Verification items for this drawing (mm, ordinates from the low corner). A direction names the side the tool comes from. Coordinates: 2 decimals unless noted, no trailing zeros. Order: outer loops, then holes, each group sorted by start corner. A loop starts at its lowest first (then second) coordinate and runs counter-clockwise, first axis right, second up.
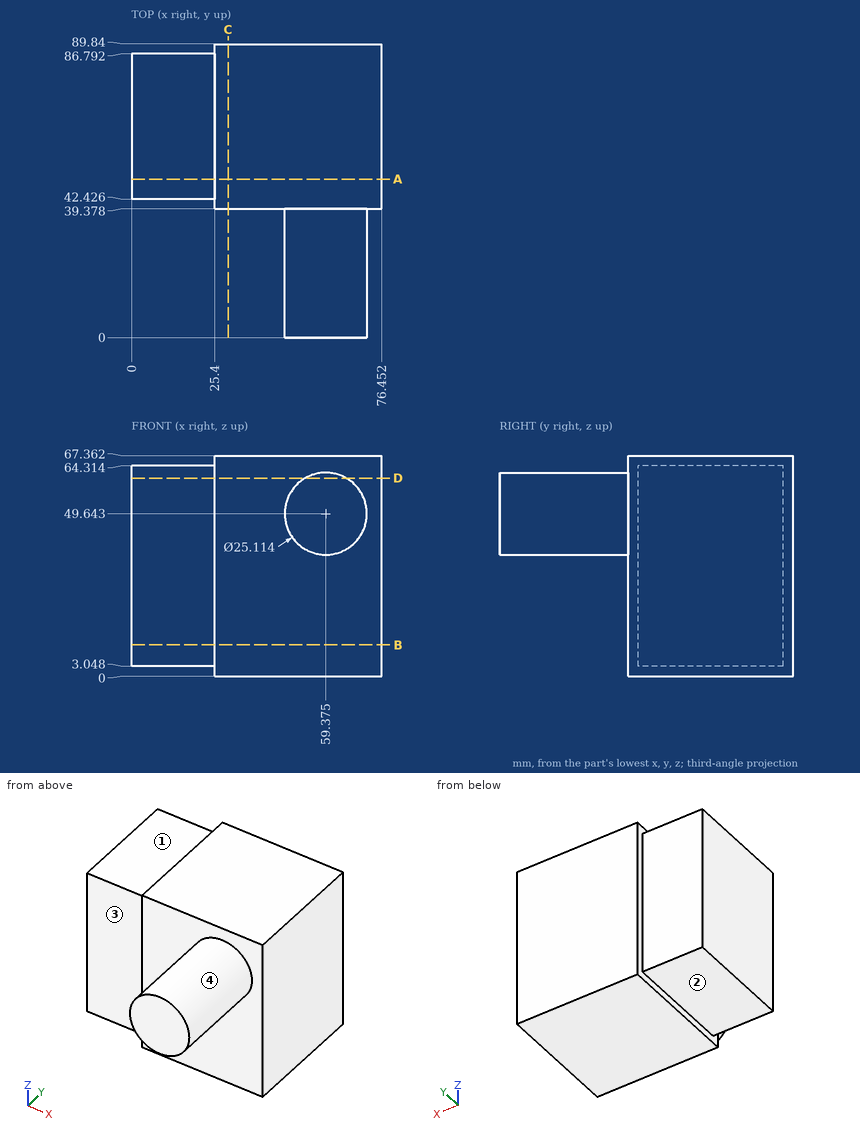
(1) Go/stop test with flat-tipped pins: P1, Ø8, axis at x = 42, y = 73, coming from the -Z side; P2, Ø7.5, axis at x = 12, z = 30, coming from the +Y side; P3, Ø3, axis at x = 38.5, z = 21.5, coming from the -Y side; P4, Ø7.5, axis at x = 14, z = 49, coming from the -Y side. Record where each tip stops, or that it passes through.
Filled in:
P1: stops at z = 0
P2: stops at y = 86.79
P3: stops at y = 39.38
P4: stops at y = 42.43
(2) Cross-section at D-D (z = 60.5). Enter the section's corners in (x, y) (1 decimal), and give its area (3 significant figures).
Filled in:
outline: (0, 42.4) - (25.4, 42.4) - (25.4, 39.4) - (53.1, 39.4) - (53.1, 0) - (65.7, 0) - (65.7, 39.4) - (76.5, 39.4) - (76.5, 89.8) - (25.4, 89.8) - (25.4, 86.8) - (0, 86.8) - close
area: 4,200 mm2
(3) Cross-section at A-A (y = 48.5). Enter the section's corners in (x, z).
Filled in:
outline: (0, 3.05) - (25.4, 3.05) - (25.4, 0) - (76.45, 0) - (76.45, 67.36) - (25.4, 67.36) - (25.4, 64.31) - (0, 64.31) - close
(4) Cross-section at C-C (x = 29.5). Enter the section's corners in (y, z), and give its area (3 significant figures).
Filled in:
outline: (39.38, 0) - (89.84, 0) - (89.84, 67.36) - (39.38, 67.36) - close
area: 3,400 mm2
(5) Thickness scan on probe 1 along Y at (x, z) = (68, 13.5); probe 2 along Y at (x, z) = (15.5, 43.5) (1 decimal); probe 3 along Z at (x, y) = (18.5, 82.5). Record the ranges inside material, lowest first.
Filled in:
probe 1: y = 39.38 to 89.84
probe 2: y = 42.4 to 86.8
probe 3: z = 3.05 to 64.31
(6) Cross-section at B-B (z = 9.5). Enter the section's corners in (x, y) (1 decimal).
Filled in:
outline: (0, 42.4) - (25.4, 42.4) - (25.4, 39.4) - (76.5, 39.4) - (76.5, 89.8) - (25.4, 89.8) - (25.4, 86.8) - (0, 86.8) - close
(7) Tool access check on the marked faces 1, 2, 3 and 4. Record the directions out of +Z, -Z, +X, -X, +Y, -Y that give a thin tool (end or side, any length) a straight path to the whole face; none if there is none.
Filled in:
face 1: +Z, -X, +Y, -Y
face 2: -Z, -X, +Y, -Y
face 3: +Z, -Z, -X, -Y
face 4: -Y
